from build123d import *

# Parameters (mm, degrees)
EXTRUDE_1_DEPTH = 15
SKETCH_2_R      = 1.25
EXTRUDE_2_DEPTH = 3
EXTRUDE_START   = 3
SKETCH_3_R      = 1.25
EXTRUDE_3_DEPTH = 3


with BuildPart() as part:
    # 草图1 → 凸台-拉伸1 (new body)
    with BuildSketch(Plane(origin=(0, 0, 0), x_dir=(1, 0, 0), z_dir=(0, 1, 0))):
        with BuildLine():
            Line((-1.25, 0), (-1.25, 7))
            ThreePointArc((-1.25, 7), (0, 8.25), (1.25, 7))
            Line((1.25, 7), (1.25, 0))
            ThreePointArc((1.25, 0), (0, -1.25), (-1.25, 0))
        make_face()
    extrude(amount=EXTRUDE_1_DEPTH)

    # 草图2 → 凸台-拉伸2 (add)
    with BuildSketch(Plane(origin=(0, 15, 0), x_dir=(1, 0, 0), z_dir=(0, 1, 0))):
        Circle(SKETCH_2_R)
    extrude(amount=EXTRUDE_2_DEPTH)

    # 草图3 → 凸台-拉伸3 (add)
    with BuildSketch(Plane.XZ.offset(EXTRUDE_START)):
        with Locations(Location((0, 0, 0), (0, 0, 270))):
            Circle(SKETCH_3_R)
    extrude(amount=-EXTRUDE_3_DEPTH)


solid = part.part
Can you work these out from the model? Positions are in its coordinate system, mm. A direction names the side the tool comes from. Give positions to 0.01 mm unless a question says otherwise; leave off trailing zeros. Loops run counter-clockwise (first coordinate to the right, second up) from the corner with the lowest first, then second, coordinate; pieces in that order, holes last. Notation, with made-up numbers: (-0.5, 43.5) - (17.5, 43.5) arc R22 cw to (17.5, 57.5) - close; hole circle Ø9 at (10, 80). An arc over 180 degrees is marked (long way). Answer as a JSON object with one key per item and string values.
Q1. Will these pins go through, and if not, where does the flat tip stop? P1, Ø1.5, axis at x = 1, z = -6, coming from the +Y side; P2, Ø1.2, axis at x = 0.5, z = -5, coming from the -Y side.
Geometry says:
{"P1": "y = 15", "P2": "y = 0"}
Q2. Imagine slicing it at C-C on y = 1. Write out the boundary of the cut face in (x, z), plus the area to 3 significant figures.
Geometry says:
{"outline": "(-1.25, -7) arc R1.25 ccw to (1.25, -7) - (1.25, 0) arc R1.25 ccw to (-1.25, 0) - close", "area": "22.4 mm²"}
Q3. Imagine slicing it at D-D on x = -0.7. Write out the boundary of the cut face in (y, z).
Geometry says:
{"outline": "(-3, -1.04) - (0, -1.04) - (0, -8.04) - (15, -8.04) - (15, -1.04) - (18, -1.04) - (18, 1.04) - (-3, 1.04) - close"}
Q4. Imagine slicing it at B-B on z = -1. Write out the boundary of the cut face in (x, y).
Geometry says:
{"outline": "(-1.25, 0) - (-0.75, 0) - (-0.75, -3) - (0.75, -3) - (0.75, 0) - (1.25, 0) - (1.25, 15) - (0.75, 15) - (0.75, 18) - (-0.75, 18) - (-0.75, 15) - (-1.25, 15) - close"}
Q5. Which directions (+Z, -Z, +X, -X, +Y, -Y) give clear straight access to the entire face, cutting with the end or side of a thin tool? Please do faces 1 (the cylindrical face through (0.177, 7.353, 1.237)), 2 (the flat face through (1.25, 7, -4)).
Geometry says:
{"face 1": "none", "face 2": "+Z, -Z, +X, +Y, -Y"}
Q6. Imagine slicing it at A-A on x = 0.45. Write out the boundary of the cut face in (y, z), plus the area to 3 significant figures.
Geometry says:
{"outline": "(-3, -1.17) - (0, -1.17) - (0, -8.17) - (15, -8.17) - (15, -1.17) - (18, -1.17) - (18, 1.17) - (-3, 1.17) - close", "area": "154 mm²"}
Q7. If I drill on L1, parallel to Z at x = 0.1, y = 9.5; L2, parallel to Y at x = 0.9, z = -1; L3, parallel to Z at x = -1.1, y = 0.25, over which ranges is the centre line in solid material (lowest first)?
Geometry says:
{"L1": "-8.25 to 1.25", "L2": "0 to 15", "L3": "-7.59 to 0.59"}
